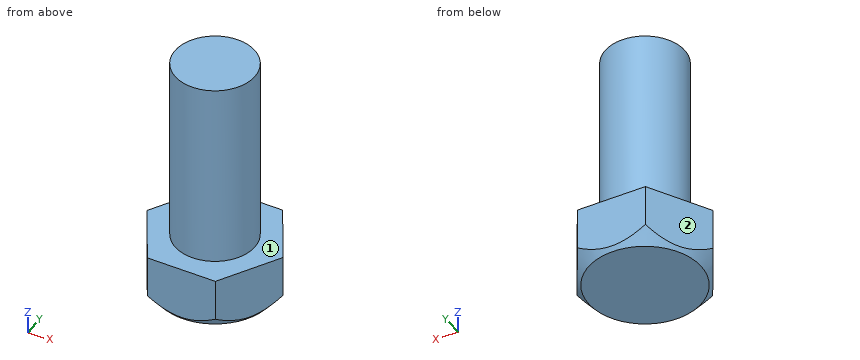
from build123d import *

# Parameters (mm, degrees)
SALIENTE_EXTRUIR1_DEPTH = 9
CROQUIS2_R              = 6.35
SALIENTE_EXTRUIR2_DEPTH = 30
CROQUIS3_R              = 18.81463578
CROQUIS3_R_2            = 9
CORTAR_EXTRUIR1_DEPTH   = 10
CORTAR_EXTRUIR1_TAPER   = 40


with BuildPart() as part:
    # Croquis1 → Saliente-Extruir1 (new body)
    with BuildSketch(Plane.XY):
        Polygon((10.969655115, 0), (5.484827557, 9.5), (-5.484827557, 9.5), (-10.969655115, 0), (-5.484827557, -9.5), (5.484827557, -9.5), align=None)
    extrude(amount=SALIENTE_EXTRUIR1_DEPTH)

    # Croquis2 → Saliente-Extruir2 (add)
    with BuildSketch(Plane.XY.offset(9)):
        Circle(CROQUIS2_R)
    extrude(amount=SALIENTE_EXTRUIR2_DEPTH)

    # Croquis3 → Cortar-Extruir1 (cut)
    with BuildSketch(Plane(origin=(0, 0, 0), x_dir=(-1, 0, 0), z_dir=(0, 0, -1))):
        Circle(CROQUIS3_R)
        Circle(CROQUIS3_R_2, mode=Mode.SUBTRACT)
    extrude(amount=-CORTAR_EXTRUIR1_DEPTH, taper=CORTAR_EXTRUIR1_TAPER, mode=Mode.SUBTRACT)


solid = part.part
Model file for the job. Use its own axes, mm. Face numbers are marked on the shaded views. A direction names the side the tool comes from. Round coordinates to 2 decimals unless told otherwise and drop trailing zeros. Loops run counter-clockwise (first coordinate to the right, second up) from the corner with the lowest first, then second, coordinate; pieces in that order, holes last. Notation, with made-up numbers: M 59.25,-19 L 97.25,-19 A17 cw 97.25,6 Z; hole C 20.25,-10.5 d4. An arc over 180 degrees is marked long. One line per question, with ' | ' between items.
1) 3-axis set-ups, long thin cutter, end or side, ignore diameter. For the marked faces 1 and 2: which of +Z, -Z, +X, -X, +Y, -Y reach the whole face in a straight line?
Solved:
face 1: +Z | face 2: +Z, -Z, -X, +Y
2) Band-saw the part on B-B (z = 5). Give the cut face in (x, y).
Solved:
outline: M -10.97,0 L -5.48,-9.5 L 5.48,-9.5 L 10.97,0 L 5.48,9.5 L -5.48,9.5 Z
3) Band-saw the part on A-A (x = 0). Give the cut face in (y, z).
Solved:
outline: M -9.5,0.6 L -9,0 L 9,0 L 9.5,0.6 L 9.5,9 L 6.35,9 L 6.35,39 L -6.35,39 L -6.35,9 L -9.5,9 Z
4) Band-saw the part on C-C (z = 18). Give the cut face in (x, y).
Solved:
outline: C 0,0 d12.7
5) Drill centre lines: line 1 along Y through (x, z) = (-0.25, 36); line 2 along Z through (x, y) = (8.25, -2); line 3 along X through (y, z) = (1, 28). Where is each one in solid material? Low to high.
Solved:
line 1: y = -6.35 to 6.35 | line 2: z = 0 to 9 | line 3: x = -6.27 to 6.27
6) Flat gauge pins, fed straight in: pin 1 (5 mm diameter, centred on x = -6.5, z = 27, fed in from -Y); pin 2 (2 mm diameter, centred on x = 7.5, z = 22.5, fed in from -Y); pin 3 (4 mm diameter, centred on x = 2.5, z = 32, fed in from +Y); pin 4 (10 mm diameter, centred on x = -5, y = -7.5, fed in from -Z). Where does each tip first touch, or does it go through?
Solved:
pin 1: stops at y = -4.93 | pin 2: passes through | pin 3: stops at y = 6.33 | pin 4: stops at z = 0
